from build123d import *

# Parameters (mm, degrees)
SKETCH1_R                = 5.375
BOSS_EXTRUDE1_DEPTH      = 3
SKETCH2_R                = 5.375
BOSS_EXTRUDE2_DEPTH      = 5
BOSS_EXTRUDE2_DRAFT      = -6
SKETCH3_R                = 5.900521176
BOSS_EXTRUDE3_DEPTH      = 32.75
BOSS_EXTRUDE4_DEPTH      = 3.5
SKETCH6_R                = 6.846847864
BOSS_EXTRUDE5_DEPTH      = 0.396875
SKETCH7_R                = 7
BOSS_EXTRUDE6_DEPTH      = 4.5
SKETCH8_R                = 7
BOSS_EXTRUDE7_DEPTH      = 3
BOSS_EXTRUDE7_TAPER      = 45
BOSS_EXTRUDE8_DEPTH      = 2
BOSS_EXTRUDE8_DEPTH_BACK = 2
SKETCH9_R                = 4.75
SKETCH9_R_2              = 1.25
FILLET1_R                = 1
FILLET2_R                = 1.5
SKETCH10_R               = 1.5
CUT_EXTRUDE1_DEPTH       = 44.25


with BuildPart() as part:
    # Sketch1 → Boss-Extrude1 (new body)
    with BuildSketch(Plane(origin=(0, 0, 0), x_dir=(1, 0, 0), z_dir=(0, 1, 0))):
        with Locations(Location((0, 0, 0), (0, 0, 270))):
            Circle(SKETCH1_R)
    extrude(amount=BOSS_EXTRUDE1_DEPTH)


with BuildPart() as boss_extrude2_tool:
    # Sketch2 → Boss-Extrude2 (with draft: the straight prism first)
    with BuildSketch(Plane(origin=(0, 3, 0), x_dir=(1, 0, 0), z_dir=(0, 1, 0))):
        with Locations(Location((0, 0, 0), (0, 0, 270))):
            Circle(SKETCH2_R)
    extrude(amount=BOSS_EXTRUDE2_DEPTH)
    # Boss-Extrude2: the draft: its side faces are tilted about the plane it starts from
    boss_extrude2_sides = [boss_extrude2_tool.faces().sort_by_distance(p)[0] for p in [
        (0, 5.5, -5.375),
    ]]
    draft(boss_extrude2_sides, Plane(origin=(0, 3, 0), x_dir=(1, 0, 0), z_dir=(0, 1, 0)), BOSS_EXTRUDE2_DRAFT)


with BuildPart() as part_1:
    add(part.part)

    # Boss-Extrude2: add boss_extrude2_tool
    add(boss_extrude2_tool.part)

    # Sketch3 → Boss-Extrude3 (add)
    with BuildSketch(Plane(origin=(0, 8, 0), x_dir=(1, 0, 0), z_dir=(0, 1, 0))):
        with Locations(Location((0, 0, 0), (0, 0, 270))):
            Circle(SKETCH3_R)
    extrude(amount=BOSS_EXTRUDE3_DEPTH)

    # Sketch5 → Boss-Extrude4 (add)
    with BuildSketch(Plane(origin=(0, 40.75, 0), x_dir=(1, 0, 0), z_dir=(0, 1, 0))):
        Polygon((-4.041451884, 7), (-8.082903769, 0), (-4.041451884, -7), (4.041451884, -7), (8.082903769, 0), (4.041451884, 7), align=None)
    extrude(amount=BOSS_EXTRUDE4_DEPTH)

    # Sketch6 → Boss-Extrude5 (add)
    with BuildSketch(Plane(origin=(0, 44.25, 0), x_dir=(1, 0, 0), z_dir=(0, 1, 0))):
        with Locations(Location((0, 0, 0), (0, 0, 270))):
            Circle(SKETCH6_R)
    extrude(amount=BOSS_EXTRUDE5_DEPTH)

    # Sketch7 → Boss-Extrude6 (add)
    with BuildSketch(Plane(origin=(0, 44.646875, 0), x_dir=(1, 0, 0), z_dir=(0, 1, 0))):
        with Locations(Location((0, 0, 0), (0, 0, 270))):
            Circle(SKETCH7_R)
    extrude(amount=BOSS_EXTRUDE6_DEPTH)

    # Sketch8 → Boss-Extrude7 (add)
    with BuildSketch(Plane(origin=(0, 49.146875, 0), x_dir=(1, 0, 0), z_dir=(0, 1, 0))):
        with Locations(Location((0, 0, 0), (0, 0, 270))):
            Circle(SKETCH8_R)
    extrude(amount=BOSS_EXTRUDE7_DEPTH, taper=BOSS_EXTRUDE7_TAPER)

    # Sketch9 → Boss-Extrude8 (add, two sides: drawn at the far end of the back side and taken through both)
    # profile 1 of 2: a face of its own
    with BuildSketch(Plane.XY.offset(-BOSS_EXTRUDE8_DEPTH_BACK)):
        with Locations((0, 54.896875)):
            Circle(SKETCH9_R)
        with Locations((0, 54.896875)):
            Circle(SKETCH9_R_2, mode=Mode.SUBTRACT)
    # profile 2 of 2: a face of its own
    with BuildSketch(Plane.XY.offset(-BOSS_EXTRUDE8_DEPTH_BACK)):
        with BuildLine():
            Line((6.179622496, 49.146875), (4.631634766, 55.950658372))
            ThreePointArc((4.631634766, 55.950658372), (4.72031594, 55.427080084), (4.75, 54.896875))
            ThreePointArc((4.75, 54.896875), (-0.530205084, 50.17655906), (-4.631634766, 55.950658372))
            Line((-4.631634766, 55.950658372), (-6.179622496, 49.146875))
            Line((-6.179622496, 49.146875), (6.179622496, 49.146875))
        make_face()
    extrude(amount=BOSS_EXTRUDE8_DEPTH + BOSS_EXTRUDE8_DEPTH_BACK)

    # Fillet1
    fillet1_edges = [part_1.edges().sort_by_distance(p)[0] for p in [
        (2, 52.146875, 3.464101615),
        (0, 49.146875, -7),
        (0, 52.146875, -4),
    ]]
    fillet(fillet1_edges, radius=FILLET1_R)

    # Fillet2
    fillet2_edges = [part_1.edges().sort_by_distance(p)[0] for p in [
        (-5.332362658, 52.870788493, -2),
        (0, 59.646875, -2),
        (-5.332362658, 52.870788493, 2),
        (0, 59.646875, 2),
        (5.332362658, 52.870788493, -2),
        (5.332362658, 52.870788493, 2),
    ]]
    fillet(fillet2_edges, radius=FILLET2_R)

    # Sketch10 → Cut-Extrude1 (cut)
    with BuildSketch(Plane.XZ):
        with Locations(Location((0, 0, 0), (0, 0, 270))):
            Circle(SKETCH10_R)
    extrude(amount=-CUT_EXTRUDE1_DEPTH, mode=Mode.SUBTRACT)


solid = part_1.part
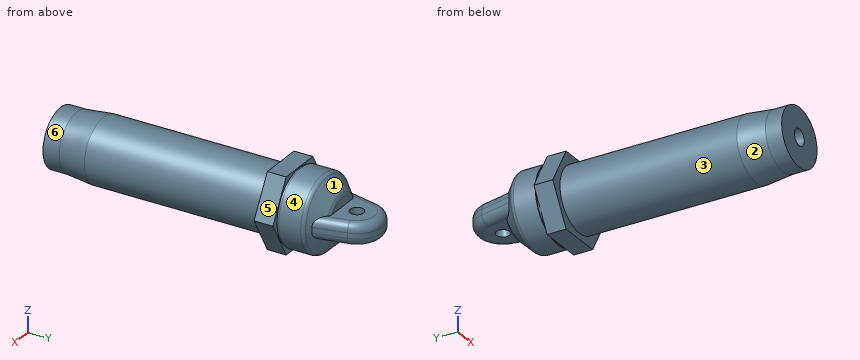
Input: part model. Units: mm. Frame: model coordinates. Face numbers are marked on the shaded views. A direction names the side the tool comes from. Give positions to 0.01 mm unless a question says otherwise; leave off trailing zeros. Order: outer loops, then holes, each group sorted by start corner. A loop starts at its lowest first (then second) coordinate and runs counter-clockwise, first axis right, second up. Notation, with made-up numbers: (79, -28.75) -> (95, -28.75) arc R20 ccw to (95, 7.25) -> close; hole circle Ø8 at (-38, 86.25). An arc over 180 degrees is marked (long way). Use one line per item in the form item = value.
1) First-contact query: pin 1 Ø4 at (x, z) = (4, 0.5) entering from +Y; pin 2 Ø1.8 at (x, z) = (0, 0) entering from -Y; pin 3 Ø0.5 at (x, z) = (0.5, 2.5) entering from +Y. Flat tips, straight axial feed; report the tip coordinate or a pass-through.
Response values:
pin_1 = 59.21
pin_2 = 44.25
pin_3 = 52.15
2) Mould query, pull axis Y, two halves, no side actions, for the marked faces 1, 2 and 3. Classes: pulls with the +Y half, pulls with the -Y half, needs draft (parallel to the pull), parting line crosses it, or undercut.
Response values:
face_1 = pulls with the +Y half
face_2 = pulls with the -Y half
face_3 = needs draft
3) Section A-A, the plane y = 18. Return loops of the section in (x, z).
Response values:
outline = circle Ø11.8 at (0, 0); hole circle Ø3 at (0, 0)
4) Line query: probe 1 along X at (y, z) = (32, 0); probe 2 along Z at (x, y) = (-3, 54.5); probe 3 along Y at (x, z) = (-2.25, -3). Output: solid intervals per line, ascending.
Response values:
probe_1 = -5.9 to -1.5, 1.5 to 5.9
probe_2 = -2 to 2
probe_3 = 0 to 52.13
5) Reachability of the marked faces 4, 5 and 6 from +Z, -Z, +X, -X, +Y, -Y: full face, straight path, thin tool, end or side. Return the list, or none.
Response values:
face_4 = +Y
face_5 = +Z, +X, +Y, -Y
face_6 = -Y
